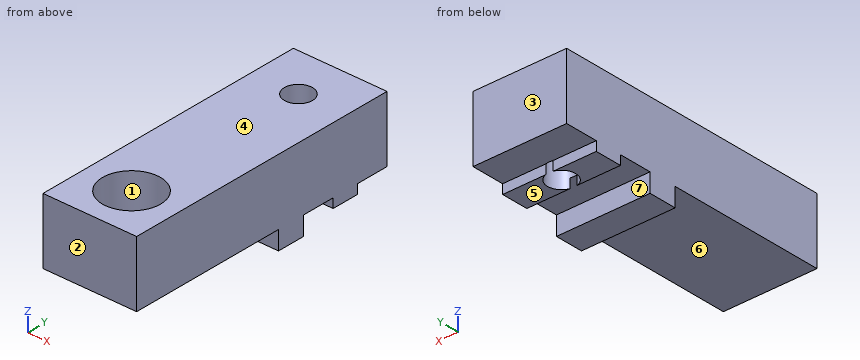
from build123d import *

# Parameters (mm, degrees)
SKETCH1_W           = 10
SKETCH1_H           = 30
MAIN_DEPTH          = 7
SKETCH2_R           = 3.1
SHAFTHOLE_DEPTH     = 4
SKETCH3_W           = 10
SKETCH3_H           = 2.9
BOSS_EXTRUDE1_DEPTH = 1
SKETCH4_R           = 1.5
CUT_EXTRUDE1_DEPTH  = 18.720045147
SKETCH5_W           = 10
SKETCH5_H           = 3
BOSS_EXTRUDE2_DEPTH = 2


with BuildPart() as part:
    # Sketch1 → Main (new body)
    with BuildSketch(Plane.XY):
        Rectangle(SKETCH1_W, SKETCH1_H)
    extrude(amount=MAIN_DEPTH)

    # Sketch2 → ShaftHole (cut)
    with BuildSketch(Plane.XY.offset(7)):
        with Locations((0, -10)):
            Circle(SKETCH2_R)
    extrude(amount=-SHAFTHOLE_DEPTH, mode=Mode.SUBTRACT)

    # Sketch3 → Boss-Extrude1 (add)
    with BuildSketch(Plane(origin=(0, 0, 0), x_dir=(-1, 0, 0), z_dir=(0, 0, -1))):
        with Locations((0, 10)):
            Rectangle(SKETCH3_W, SKETCH3_H)
    extrude(amount=BOSS_EXTRUDE1_DEPTH)

    # Sketch4 → Cut-Extrude1 (cut, through all)
    with BuildSketch(Plane.XY.offset(7)):
        with Locations((0, 10)):
            Circle(SKETCH4_R)
    extrude(amount=-CUT_EXTRUDE1_DEPTH, mode=Mode.SUBTRACT)

    # Sketch5 → Boss-Extrude2 (add)
    with BuildSketch(Plane(origin=(0, 0, 0), x_dir=(-1, 0, 0), z_dir=(0, 0, -1))):
        with Locations((0, 3.5)):
            Rectangle(SKETCH5_W, SKETCH5_H)
    extrude(amount=BOSS_EXTRUDE2_DEPTH)


solid = part.part
Geometry: final body of the model. Coordinates: model frame, mm. Face numbers are marked on the shaded views. A direction names the side the tool comes from. Round coordinates to 2 decimals unless told otherwise and drop trailing zeros. Write each loop counter-clockwise with the first axis right and the second up, starting at its lowest first coordinate (ties: lowest second). Pieces come first, ordered by that corner, then holes. Notation, with made-up numbers: M 42,-9 L 57,-9 A29 ccw 57,28 Z; hole C 74.5,38 d8. An arc over 180 degrees is marked long. Write item = value, one per line.
Item 1: Pull-direction query (Y, two-part tool) for the marked faces 1, 2, 3 and 4; classes: pulls with the +Y half, pulls with the -Y half, needs draft (parallel to the pull), parting line crosses it, or undercut.
Findings:
face_1 = undercut
face_2 = pulls with the -Y half
face_3 = pulls with the +Y half
face_4 = needs draft
Item 2: Section query B-B on x = 0. Return loops of the section in (y, z), then the cut area to 3 significant figures.
Findings:
outline = M -15,0 L 2,0 L 2,-2 L 5,-2 L 5,0 L 8.5,0 L 8.5,7 L -6.9,7 L -6.9,3 L -13.1,3 L -13.1,7 L -15,7 Z; M 11.5,0 L 15,0 L 15,7 L 11.5,7 Z
area = 170 mm^2
Item 3: Pin query (flat end, axial travel): P1, Ø2, axis at x = -1, z = -1.5, coming from the +Y side; P2, Ø2.5, axis at x = 2.5, y = 10, coming from the -Z side; P3, Ø1, axis at x = -0.5, z = -1, coming from the -Y side. Return the tip coordinate at first contact, or that it passes through.
Findings:
P1 = 11.45
P2 = -1
P3 = 2
Item 4: Section query D-D on x = 4.25. Return loops of the section in (y, z).
Findings:
outline = M -15,0 L 2,0 L 2,-2 L 5,-2 L 5,0 L 8.55,0 L 8.55,-1 L 11.45,-1 L 11.45,0 L 15,0 L 15,7 L -15,7 Z
Item 5: Material intervals for line 1 along Y through (x, z) = (0, 4.75); line 2 along X through (y, z) = (10, 4); line 3 along Y through (x, z) = (-1, 3.5), sorted ascending. Write a range as [from, to].
Findings:
line_1 = [-15, -13.1], [-6.9, 8.5], [11.5, 15]
line_2 = [-5, -1.5], [1.5, 5]
line_3 = [-15, -12.93], [-7.07, 8.88], [11.12, 15]
Item 6: Access query for the marked faces 5, 6 and 7. Directions: +Z, -Z, +X, -X, +Y, -Y. A direction counts if a zero-diameter tool reaches every point of the face in a straight line with its end or side. Return the directions, or none.
Findings:
face_5 = -Z, +X, -X, +Y
face_6 = -Z, +X, -X, -Y
face_7 = -Z, +X, -X
Item 7: Section query C-C on z = 4.25. Return loops of the section in (x, y), then the cut area to 3 significant figures.
Findings:
outline = M -5,-15 L 5,-15 L 5,15 L -5,15 Z; hole C 0,-10 d6.2; hole C 0,10 d3
area = 263 mm^2
Item 8: Section query A-A on y = 10. Return loops of the section in (x, z), then the cut area to 3 significant figures.
Findings:
outline = M -5,-1 L -1.5,-1 L -1.5,7 L -5,7 Z; M 1.5,-1 L 5,-1 L 5,7 L 1.5,7 Z
area = 56.0 mm^2
